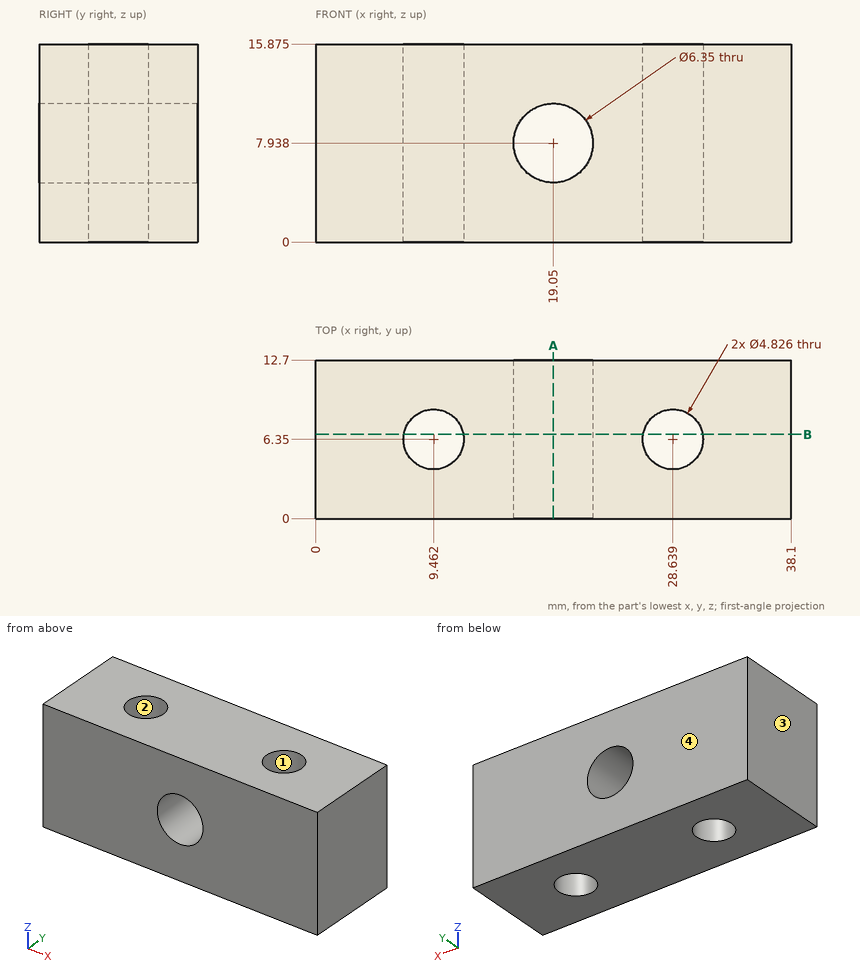
Study the drawing (mm; zero at the part's minimum x, y, z) and answer. Coordinates: 2 decimals unless noted, no trailing zeros. Write each loop counter-clockwise with the first axis right and the second up, starting at its lowest first coordinate (ties: lowest second). Pieces come first, ordered by that corner, then holes.
Q1. A cutting plane is placed at A-A, the plane x = 19.05. Give the vertices of the cut face in (y, z) (1 decimal), then the cut area to 3 significant figures.
Q2. A cutting plane is placed at B-B, the plane y = 6.75. State how many separate pieces and enclosed holes the cut face has, then the cut area to 3 significant figures.
Q3. Determine the mould class of the marked faces 1, 2, 3 and 4 for opening direction Y: released by +Y, released by -Y, zero draft, split by the parting line, or undercut.
Q4. Find the intervals of material crossed by line 1 (X direction, y = 4.75, z = 13.5) (1 decimal); line 2 (X direction, y = 5.5, z = 8) (1 decimal); line 3 (X direction, y = 3.5, z = 10.75) (1 decimal), in increasing order.
Findings below:
1. outline: (0, 0) - (12.7, 0) - (12.7, 4.8) - (0, 4.8) - close; (0, 11.1) - (12.7, 11.1) - (12.7, 15.9) - (0, 15.9) - close
1. area: 121 mm2
2. separate pieces: 3
2. enclosed holes: 1
2. area: 422 mm2
3. face 1: undercut
3. face 2: undercut
3. face 3: zero draft
3. face 4: released by +Y
4. line 1: x = 0 to 7.7, 11.3 to 26.8, 30.4 to 38.1
4. line 2: x = 0 to 7.2, 11.7 to 15.9, 22.2 to 26.4, 30.9 to 38.1
4. line 3: x = 0 to 17.6, 20.5 to 38.1
